Could you check a few things on this model? Use its own coordinates, in mm. Coordinates: 2 decimals unless noted, no trailing zeros. Return JSON: item names as keys, results as strings. Group by question number.
from build123d import *

# Parameters (mm, degrees)
SKETCH1_W           = 140
SKETCH1_H           = 140
SKETCH1_R           = 1.65
SKETCH1_R_2         = 1.5
SKETCH1_W_2         = 3.175
SKETCH1_H_2         = 12
SKETCH1_W_3         = 12
SKETCH1_H_3         = 3.175
SKETCH1_W_4         = 18
SKETCH1_H_4         = 1
BOSS_EXTRUDE1_DEPTH = 3.175
FILLET1_R           = 10


with BuildPart() as part:
    # Sketch1 → Boss-Extrude1 (new body)
    with BuildSketch(Plane(origin=(0, 0, 0), x_dir=(1, 0, 0), z_dir=(0, 1, 0))):
        Rectangle(SKETCH1_W, SKETCH1_H)
        with Locations((62.928932188, -62.928932188)):
            Circle(SKETCH1_R, mode=Mode.SUBTRACT)
        with Locations((62.928932188, 62.928932188)):
            Circle(SKETCH1_R, mode=Mode.SUBTRACT)
        with Locations((-62.928932188, -62.928932188)):
            Circle(SKETCH1_R, mode=Mode.SUBTRACT)
        with Locations((-62.928932188, 62.928932188)):
            Circle(SKETCH1_R, mode=Mode.SUBTRACT)
        with Locations((7, 52.65)):
            Circle(SKETCH1_R_2, mode=Mode.SUBTRACT)
        with Locations((-7, 52.65)):
            Circle(SKETCH1_R_2, mode=Mode.SUBTRACT)
        with Locations((-65.2375, -14)):
            Rectangle(SKETCH1_W_2, SKETCH1_H_2, mode=Mode.SUBTRACT)
        with Locations((65.2375, -14)):
            Rectangle(SKETCH1_W_2, SKETCH1_H_2, mode=Mode.SUBTRACT)
        with Locations((14, -65.2375)):
            Rectangle(SKETCH1_W_3, SKETCH1_H_3, mode=Mode.SUBTRACT)
        with Locations((-14, -65.2375)):
            Rectangle(SKETCH1_W_3, SKETCH1_H_3, mode=Mode.SUBTRACT)
        with Locations((65.2375, 14)):
            Rectangle(SKETCH1_W_2, SKETCH1_H_2, mode=Mode.SUBTRACT)
        with Locations((14, 65.2375)):
            Rectangle(SKETCH1_W_3, SKETCH1_H_3, mode=Mode.SUBTRACT)
        with Locations((-14, 65.2375)):
            Rectangle(SKETCH1_W_3, SKETCH1_H_3, mode=Mode.SUBTRACT)
        with Locations((-65.2375, 14)):
            Rectangle(SKETCH1_W_2, SKETCH1_H_2, mode=Mode.SUBTRACT)
        with Locations((0, 61.15)):
            Rectangle(SKETCH1_W_4, SKETCH1_H_4, mode=Mode.SUBTRACT)
    extrude(amount=BOSS_EXTRUDE1_DEPTH)

    # Fillet1
    fillet1_edges = [part.edges().sort_by_distance(p)[0] for p in [
        (70, 1.5875, 70),
        (-70, 1.5875, 70),
        (-70, 1.5875, -70),
        (70, 1.5875, -70),
    ]]
    fillet(fillet1_edges, radius=FILLET1_R)


solid = part.part
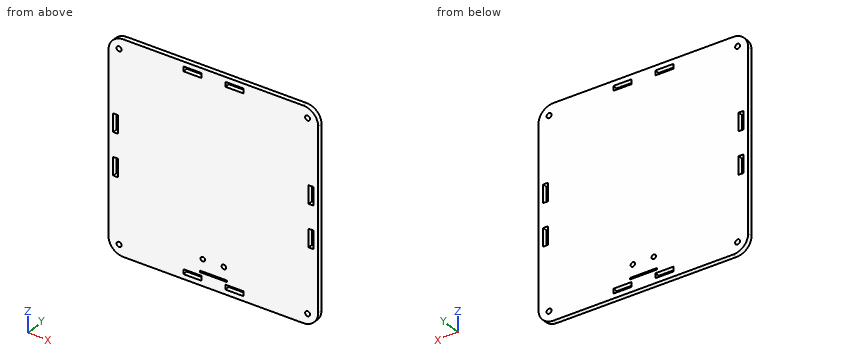
(1) If I drill on L1, parallel to X at y = 0.5, z = -13.5 (3 decimals); L2, parallel to Z at x = 7, y = 2, over which ranges is the centre line in solid material (lowest first)? Write a range as [from, to].
(2) Will these pins go through, and if not, where does the flat tip stop? P1, Ø2.5, axis at x = 7, z = -52.65, coming from the -Y side; P2, Ø1, axis at x = 65.5, y = 2, coming from the -Z side; P3, Ø1, axis at y = 2, z = 65, coming from the -X side.
(3) Imagine slicing it at A-A, the plane y = 0.8. Count the separate pieces of the cut face and the enclosed holes in it, then the cut area to 3 significant figures.
Checks:
{
 "1": {"L1": "[-70, -66.825], [-63.65, 63.65], [66.825, 70]", "L2": "[-70, -61.65], [-60.65, -54.15], [-51.15, 70]"},
 "2": {"P1": "through", "P2": "z = -68.66", "P3": "x = -68.93"},
 "3": {"separate pieces": "1", "enclosed holes": "15", "area": "19,100 mm²"}
}
